from build123d import *

# Parameters (mm, degrees)
EXTRUDE_1_DEPTH            = 10
HOLE_WIZARD_M4_D           = 4.5
HOLE_WIZARD_M4_CBORE_D     = 8
HOLE_WIZARD_M4_CBORE_DEPTH = 4
HOLE_WIZARD_1_4_201_D      = 5.1054
HOLE_WIZARD_3_8_161_D      = 7.9375
CUT_EXTRUDE_1_DEPTH        = 11
SKETCH_14_W                = 20.2
SKETCH_14_H                = 40
CUT_EXTRUDE_2_DEPTH        = 7
SKETCH_15_R                = 2
CUT_EXTRUDE_3_DEPTH        = 7
CUT_EXTRUDE_4_DEPTH        = 11
CUT_EXTRUDE_7_DEPTH        = 5
CUT_EXTRUDE_8_DEPTH        = 5
SKETCH_18_W                = 12.9
SKETCH_18_H                = 40
CUT_EXTRUDE_6_DEPTH        = 5
FILLET_1_R                 = 3


with BuildPart() as part:
    # Эскиз1 → Бобышка-Вытянуть1 (new body)
    with BuildSketch(Plane.XY):
        Polygon((0, 0), (60, 0), (60, -60), (60, -150), (60, -190), (0, -190), align=None)
    extrude(amount=EXTRUDE_1_DEPTH)

    # Цековка для винта с внутренним шестигранником M4 (through all)
    with Locations(Plane(origin=(-14.842707118, -41.655134189, 0), x_dir=(-1, 0, 0), z_dir=(0, 0, -1))):
        with Locations((-67.342707118, 36.655134189), (-52.342707118, 36.655134189), (-37.342707118, 36.655134189), (-22.342707118, 36.655134189)):
            CounterBoreHole(HOLE_WIZARD_M4_D / 2, HOLE_WIZARD_M4_CBORE_D / 2, HOLE_WIZARD_M4_CBORE_DEPTH)

    # Отверстие обработанное метчиком 1/4-201 (through all)
    with Locations(Plane(origin=(39.25, -175, 10), x_dir=(1, 0, 0), z_dir=(0, 0, 1))):
        with Locations((0, 0)):
            Hole(HOLE_WIZARD_1_4_201_D / 2)

    # Отверстие обработанное метчиком 3/8-161 (through all)
    with Locations(Plane(origin=(21, -175, 10), x_dir=(1, 0, 0), z_dir=(0, 0, 1))):
        with Locations((0, 0)):
            Hole(HOLE_WIZARD_3_8_161_D / 2)

    # Эскиз12 → Вырез-Вытянуть1 (cut, through all)
    with BuildSketch(Plane.XY.offset(10)):
        with BuildLine():
            Line((36.75, -175), (36.75, -70))
            ThreePointArc((36.75, -70), (39.25, -67.5), (41.75, -70))
            Line((41.75, -70), (41.75, -175))
            ThreePointArc((41.75, -175), (39.25, -177.5), (36.75, -175))
        make_face()
        with BuildLine():
            Line((18.5, -175), (18.5, -70))
            ThreePointArc((18.5, -70), (21, -67.5), (23.5, -70))
            Line((23.5, -70), (23.5, -175))
            ThreePointArc((23.5, -175), (21, -177.5), (18.5, -175))
        make_face()
    extrude(amount=-CUT_EXTRUDE_1_DEPTH, mode=Mode.SUBTRACT)

    # Эскиз14 → Вырез-Вытянуть2 (cut)
    with BuildSketch(Plane(origin=(0, 0, 0), x_dir=(-1, 0, 0), z_dir=(0, 0, -1))):
        with Locations((-30, -35)):
            Rectangle(SKETCH_14_W, SKETCH_14_H)
    extrude(amount=-CUT_EXTRUDE_2_DEPTH, mode=Mode.SUBTRACT)

    # Эскиз15 → Вырез-Вытянуть3 (cut)
    with BuildSketch(Plane(origin=(0, 0, 0), x_dir=(-1, 0, 0), z_dir=(0, 0, -1))):
        with Locations((-39.1, -54)):
            Circle(SKETCH_15_R)
        with Locations((-20.9, -54)):
            Circle(SKETCH_15_R)
    extrude(amount=-CUT_EXTRUDE_3_DEPTH, mode=Mode.SUBTRACT)

    # Эскиз16 → Вырез-Вытянуть4 (cut, through all)
    with BuildSketch(Plane(origin=(0, 0, 0), x_dir=(-1, 0, 0), z_dir=(0, 0, -1))):
        with BuildLine():
            Line((0, -180), (0, -195))
            Line((0, -195), (-60, -195))
            Line((-60, -195), (-60, -180))
            ThreePointArc((-60, -180), (-30, -190), (0, -180))
        make_face()
    extrude(amount=-CUT_EXTRUDE_4_DEPTH, mode=Mode.SUBTRACT)

    # Эскиз19 → Вырез-Вытянуть7 (cut)
    with BuildSketch(Plane(origin=(0, 0, 0), x_dir=(-1, 0, 0), z_dir=(0, 0, -1))):
        with BuildLine():
            Line((-57, -61), (-57, -177.416573868))
            ThreePointArc((-57, -177.416573868), (-55, -179.416573868), (-53, -177.416573868))
            Line((-53, -177.416573868), (-53, -61))
            ThreePointArc((-53, -61), (-55, -59), (-57, -61))
        make_face()
        with BuildLine():
            Line((-7, -61), (-7, -177.416573868))
            ThreePointArc((-7, -177.416573868), (-5, -179.416573868), (-3, -177.416573868))
            Line((-3, -177.416573868), (-3, -61))
            ThreePointArc((-3, -61), (-5, -59), (-7, -61))
        make_face()
    extrude(amount=-CUT_EXTRUDE_7_DEPTH, mode=Mode.SUBTRACT)

    # Эскиз20 → Вырез-Вытянуть8 (cut)
    with BuildSketch(Plane(origin=(0, 0, 0), x_dir=(-1, 0, 0), z_dir=(0, 0, -1))):
        with BuildLine():
            Line((-50, -59), (-50, -182.532340636))
            ThreePointArc((-50, -182.532340636), (-30, -187), (-10, -182.532340636))
            Line((-10, -182.532340636), (-10, -59))
            Line((-10, -59), (-50, -59))
        make_face()
    extrude(amount=-CUT_EXTRUDE_8_DEPTH, mode=Mode.SUBTRACT)

    # Эскиз18 → Вырез-Вытянуть6 (cut)
    with BuildSketch(Plane(origin=(0, 0, 0), x_dir=(-1, 0, 0), z_dir=(0, 0, -1))):
        with Locations((-50.55, -35)):
            Rectangle(SKETCH_18_W, SKETCH_18_H)
        with Locations((-9.45, -35)):
            Rectangle(SKETCH_18_W, SKETCH_18_H)
    extrude(amount=-CUT_EXTRUDE_6_DEPTH, mode=Mode.SUBTRACT)

    # Скругление1
    fillet_1_edges = [part.edges().sort_by_distance(p)[0] for p in [
        (19.9, -15, 3.5),
        (40.1, -15, 3.5),
        (37.367949192, -55, 3.5),
        (40.1, -52.267949192, 3.5),
        (19.9, -52.267949192, 3.5),
        (22.632050808, -55, 3.5),
        (50, -59, 2.5),
        (10, -59, 2.5),
        (10, -182.532340636, 2.5),
        (50, -182.532340636, 2.5),
        (57, -55, 2.5),
        (57, -15, 2.5),
        (44.1, -15, 2.5),
        (44.1, -55, 2.5),
        (15.9, -15, 2.5),
        (3, -15, 2.5),
        (3, -55, 2.5),
        (15.9, -55, 2.5),
    ]]
    fillet(fillet_1_edges, radius=FILLET_1_R)


solid = part.part
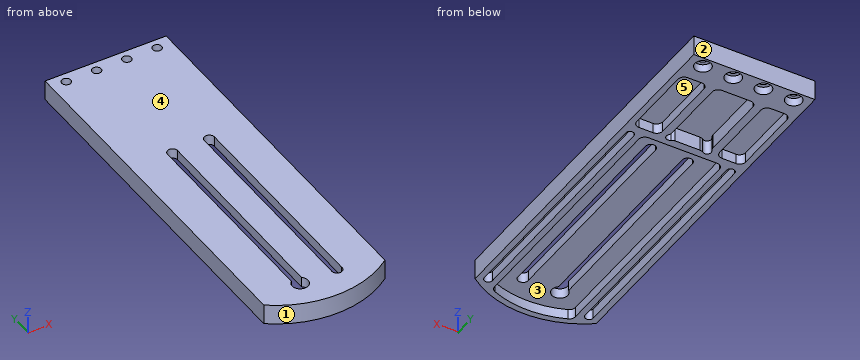
Input: part model. Units: mm. Frame: model coordinates. Face numbers are marked on the shaded views. A direction names the side the tool comes from. Round coordinates to 2 decimals unless told otherwise and drop trailing zeros. Order: outer loops, then holes, each group sorted by start corner. A loop starts at its lowest first (then second) coordinate and runs counter-clockwise, first axis right, second up. Notation, with made-up numbers: (88.25, 19) - (121.25, 19) arc R27 ccw to (121.25, 46) - close; hole circle Ø10 at (61, 70). An arc over 180 degrees is marked (long way). Answer as a JSON object with one key per item and string values. Group by question number.
(1) Cut plane A-A (y = -84). Return loops of the section in (x, z), then the cut area to 3 significant figures.
(2) Draft query along Y for the marked faces 1, 2 and 3. Return one class per face: released by +Y, released by -Y, zero draft, split by the parting line, or undercut.
(3) Cut plane B-B (y = -5). Count the separate pieces of the cut face and the enclosed holes in it, then the cut area to 3 significant figures.
(4) Reachability of the marked faces 4 and 5 from +Z, -Z, +X, -X, +Y, -Y: full face, straight path, thin tool, end or side. Return the list, or none.
(5) Material intervals for probe 1 along X at (y, z) = (-84, 1.75); probe 2 along X at (y, z) = (-153.5, 8); probe 3 along Y at (x, z) = (39.25, 8.9), sorted ascending. Write a range as from..to.
(6) Pin query (flat end, axial travel): P1, Ø4, axis at x = 22.5, y = -5, coming from the -Z side; P2, Ø3, axis at x = 48, z = 1, coming from the -Y side; P3, Ø1, axis at x = 26.5, y = -142.5, coming from the -Z side; P4, Ø4, axis at x = 44.5, z = 7, coming from the -Y side. Return the tip coordinate at first contact, or that it passes through.
Here are the results:
{
 "1": {"outline": "(0, 0) - (3, 0) - (3, 5) - (7, 5) - (7, 0) - (10, 0) - (10, 5) - (18.5, 5) - (18.5, 10) - (0, 10) - close; (23.5, 5) - (36.75, 5) - (36.75, 10) - (23.5, 10) - close; (41.75, 5) - (50, 5) - (50, 0) - (53, 0) - (53, 5) - (57, 5) - (57, 0) - (60, 0) - (60, 10) - (41.75, 10) - close", "area": "310 mm^2"},
 "2": {"face 1": "released by -Y", "face 2": "released by +Y", "face 3": "undercut"},
 "3": {"separate pieces": "5", "enclosed holes": "0", "area": "364 mm^2"},
 "4": {"face 4": "+Z, +X, -X, +Y, -Y", "face 5": "-Z"},
 "5": {"probe 1": "x = 0..3, 7..10, 50..53, 57..60", "probe 2": "x = 0..18.5, 23.5..36.75, 41.75..60", "probe 3": "y = -189.14..-177.55, -67.5..-6.41, -3.59..0"},
 "6": {"P1": "passes through", "P2": "stops at y = -187.2", "P3": "stops at z = 5", "P4": "stops at y = -188.41"}
}
